Check sheet for the modelled part. Datum: model origin and axes. Units: mm. Give positions to 0.01 mm unless a question says otherwise; leave off trailing zeros. Loops run counter-clockwise (first coordinate to the right, second up) from the corner with the lowest first, then second, coordinate; pieces in that order, holes last. Notation, with made-up numbers: (21, 81.25) - (40, 81.25) arc R23 ccw to (40, 114.25) - close; hole circle Ø11 at (-16, 82). An arc over 180 degrees is marked (long way). Use one line per item in the form item = value.
from build123d import *

# Parameters (mm, degrees)
SKETCH1_W           = 420
SKETCH1_H           = 100
SKETCH1_R           = 20
SKETCH1_R_2         = 7.5
SKETCH1_R_3         = 1.5
SKETCH1_W_2         = 5
SKETCH1_H_2         = 5
BOSS_EXTRUDE1_DEPTH = 5
FILLET1_R           = 5


with BuildPart() as part:
    # Sketch1 → Boss-Extrude1 (new body)
    with BuildSketch(Plane.XY):
        Rectangle(SKETCH1_W, SKETCH1_H)
        Circle(SKETCH1_R, mode=Mode.SUBTRACT)
        with Locations((-40, 0)):
            Circle(SKETCH1_R_2, mode=Mode.SUBTRACT)
        with Locations(Location((40, 0, 0), (0, 0, 180))):
            Circle(SKETCH1_R_2, mode=Mode.SUBTRACT)
        with Locations((0, -42.5)):
            Circle(SKETCH1_R_3, mode=Mode.SUBTRACT)
        with Locations((-54, -42.5)):
            Circle(SKETCH1_R_3, mode=Mode.SUBTRACT)
        with Locations((-108, -42.5)):
            Circle(SKETCH1_R_3, mode=Mode.SUBTRACT)
        with Locations((-162, -42.5)):
            Circle(SKETCH1_R_3, mode=Mode.SUBTRACT)
        with Locations((-202.5, 25)):
            Circle(SKETCH1_R_3, mode=Mode.SUBTRACT)
        with Locations(Location((54, -42.5, 0), (0, 0, 180))):
            Circle(SKETCH1_R_3, mode=Mode.SUBTRACT)
        with Locations(Location((108, -42.5, 0), (0, 0, 180))):
            Circle(SKETCH1_R_3, mode=Mode.SUBTRACT)
        with Locations(Location((162, -42.5, 0), (0, 0, 180))):
            Circle(SKETCH1_R_3, mode=Mode.SUBTRACT)
        with Locations(Location((-54, 42.5, 0), (0, 0, 90))):
            Circle(SKETCH1_R_3, mode=Mode.SUBTRACT)
        with Locations((162, 42.5)):
            Circle(SKETCH1_R_3, mode=Mode.SUBTRACT)
        with Locations(Location((-108, 42.5, 0), (0, 0, 90))):
            Circle(SKETCH1_R_3, mode=Mode.SUBTRACT)
        with Locations(Location((0, 42.5, 0), (0, 0, 90))):
            Circle(SKETCH1_R_3, mode=Mode.SUBTRACT)
        with Locations(Location((-162, 42.5, 0), (0, 0, 90))):
            Circle(SKETCH1_R_3, mode=Mode.SUBTRACT)
        with Locations((54, 42.5)):
            Circle(SKETCH1_R_3, mode=Mode.SUBTRACT)
        with Locations((108, 42.5)):
            Circle(SKETCH1_R_3, mode=Mode.SUBTRACT)
        with Locations(Location((-202.5, -25, 0), (0, 0, 90))):
            Circle(SKETCH1_R_3, mode=Mode.SUBTRACT)
        with Locations(Location((202.5, 25, 0), (0, 0, 180))):
            Circle(SKETCH1_R_3, mode=Mode.SUBTRACT)
        with Locations((202.5, -25)):
            Circle(SKETCH1_R_3, mode=Mode.SUBTRACT)
        with Locations((-7.5, -42.5)):
            Rectangle(SKETCH1_W_2, SKETCH1_H_2, mode=Mode.SUBTRACT)
        with Locations((7.5, -42.5)):
            Rectangle(SKETCH1_W_2, SKETCH1_H_2, mode=Mode.SUBTRACT)
        with Locations((-61.5, -42.5)):
            Rectangle(SKETCH1_W_2, SKETCH1_H_2, mode=Mode.SUBTRACT)
        with Locations((-46.5, -42.5)):
            Rectangle(SKETCH1_W_2, SKETCH1_H_2, mode=Mode.SUBTRACT)
        with Locations((-115.5, -42.5)):
            Rectangle(SKETCH1_W_2, SKETCH1_H_2, mode=Mode.SUBTRACT)
        with Locations((-100.5, -42.5)):
            Rectangle(SKETCH1_W_2, SKETCH1_H_2, mode=Mode.SUBTRACT)
        with Locations((-169.5, -42.5)):
            Rectangle(SKETCH1_W_2, SKETCH1_H_2, mode=Mode.SUBTRACT)
        with Locations((-154.5, -42.5)):
            Rectangle(SKETCH1_W_2, SKETCH1_H_2, mode=Mode.SUBTRACT)
        with Locations((-202.5, 17.5)):
            Rectangle(SKETCH1_W_2, SKETCH1_H_2, mode=Mode.SUBTRACT)
        with Locations((-202.5, 32.5)):
            Rectangle(SKETCH1_W_2, SKETCH1_H_2, mode=Mode.SUBTRACT)
        with Locations((61.5, -42.5)):
            Rectangle(SKETCH1_W_2, SKETCH1_H_2, mode=Mode.SUBTRACT)
        with Locations((46.5, -42.5)):
            Rectangle(SKETCH1_W_2, SKETCH1_H_2, mode=Mode.SUBTRACT)
        with Locations((115.5, -42.5)):
            Rectangle(SKETCH1_W_2, SKETCH1_H_2, mode=Mode.SUBTRACT)
        with Locations((100.5, -42.5)):
            Rectangle(SKETCH1_W_2, SKETCH1_H_2, mode=Mode.SUBTRACT)
        with Locations((169.5, -42.5)):
            Rectangle(SKETCH1_W_2, SKETCH1_H_2, mode=Mode.SUBTRACT)
        with Locations((154.5, -42.5)):
            Rectangle(SKETCH1_W_2, SKETCH1_H_2, mode=Mode.SUBTRACT)
        with Locations((-61.5, 42.5)):
            Rectangle(SKETCH1_W_2, SKETCH1_H_2, mode=Mode.SUBTRACT)
        with Locations((-46.5, 42.5)):
            Rectangle(SKETCH1_W_2, SKETCH1_H_2, mode=Mode.SUBTRACT)
        with Locations((169.5, 42.5)):
            Rectangle(SKETCH1_W_2, SKETCH1_H_2, mode=Mode.SUBTRACT)
        with Locations((154.5, 42.5)):
            Rectangle(SKETCH1_W_2, SKETCH1_H_2, mode=Mode.SUBTRACT)
        with Locations((-115.5, 42.5)):
            Rectangle(SKETCH1_W_2, SKETCH1_H_2, mode=Mode.SUBTRACT)
        with Locations((-100.5, 42.5)):
            Rectangle(SKETCH1_W_2, SKETCH1_H_2, mode=Mode.SUBTRACT)
        with Locations((-7.5, 42.5)):
            Rectangle(SKETCH1_W_2, SKETCH1_H_2, mode=Mode.SUBTRACT)
        with Locations((7.5, 42.5)):
            Rectangle(SKETCH1_W_2, SKETCH1_H_2, mode=Mode.SUBTRACT)
        with Locations((-169.5, 42.5)):
            Rectangle(SKETCH1_W_2, SKETCH1_H_2, mode=Mode.SUBTRACT)
        with Locations((-154.5, 42.5)):
            Rectangle(SKETCH1_W_2, SKETCH1_H_2, mode=Mode.SUBTRACT)
        with Locations((61.5, 42.5)):
            Rectangle(SKETCH1_W_2, SKETCH1_H_2, mode=Mode.SUBTRACT)
        with Locations((46.5, 42.5)):
            Rectangle(SKETCH1_W_2, SKETCH1_H_2, mode=Mode.SUBTRACT)
        with Locations((115.5, 42.5)):
            Rectangle(SKETCH1_W_2, SKETCH1_H_2, mode=Mode.SUBTRACT)
        with Locations((100.5, 42.5)):
            Rectangle(SKETCH1_W_2, SKETCH1_H_2, mode=Mode.SUBTRACT)
        with Locations((-202.5, -17.5)):
            Rectangle(SKETCH1_W_2, SKETCH1_H_2, mode=Mode.SUBTRACT)
        with Locations((-202.5, -32.5)):
            Rectangle(SKETCH1_W_2, SKETCH1_H_2, mode=Mode.SUBTRACT)
        with Locations((202.5, 17.5)):
            Rectangle(SKETCH1_W_2, SKETCH1_H_2, mode=Mode.SUBTRACT)
        with Locations((202.5, 32.5)):
            Rectangle(SKETCH1_W_2, SKETCH1_H_2, mode=Mode.SUBTRACT)
        with Locations((202.5, -17.5)):
            Rectangle(SKETCH1_W_2, SKETCH1_H_2, mode=Mode.SUBTRACT)
        with Locations((202.5, -32.5)):
            Rectangle(SKETCH1_W_2, SKETCH1_H_2, mode=Mode.SUBTRACT)
    extrude(amount=BOSS_EXTRUDE1_DEPTH)

    # Fillet1
    fillet1_edges = [part.edges().sort_by_distance(p)[0] for p in [
        (210, -50, 2.5),
        (-210, -50, 2.5),
        (-210, 50, 2.5),
        (210, 50, 2.5),
    ]]
    fillet(fillet1_edges, radius=FILLET1_R)


solid = part.part
Item 1: Section check A-A on y = 11. Record the boundary of the cut face in (x, z).
Answer block:
outline = (-210, 0) - (-16.7, 0) - (-16.7, 5) - (-210, 5) - close; (16.7, 0) - (210, 0) - (210, 5) - (16.7, 5) - close
Item 2: Section check B-B on z = 0.95. Give the number of separate pieces and of enclosed holes in the cut face, then the cut area to 3 significant figures.
Answer block:
separate_pieces = 1
enclosed_holes = 57
area = 39,300 mm2
Item 3: Mould release check, pull along Y, two halves, no side actions. Record for faces 1 (the face through (-32.846, 2.253, 2.465)), 2 (the face through (-4.336, -19.524, 2.465)), 3 (the face through (-3, 23, 5)): released by +Y, released by -Y, zero draft, split by the parting line, or undercut.
Answer block:
face_1 = undercut
face_2 = undercut
face_3 = zero draft
Item 4: Gauge pin test, flat end, axial feed: P1, Ø2.5, axis at x = -108, y = -42.5, coming from the +Z side. Record the tip position at first contact, or that the pin passes through.
Answer block:
P1 = through
Item 5: Thickness scan on L1, parallel to Y at x = 108, z = 3; L2, parallel to X at y = 32, z = 3.15; L3, parallel to Y at x = -54.5, z = 0.65. Record the ranges inside material, lowest first.
Answer block:
L1 = -50 to -44, -41 to 41, 44 to 50
L2 = -210 to -205, -200 to 200, 205 to 210
L3 = -50 to -43.91, -41.09 to 41.09, 43.91 to 50
